```python
from build123d import *

# Parameters (mm, degrees)
SKETCH2_W           = 23
SKETCH2_H           = 10
SKETCH2_R           = 1.05
BOSS_EXTRUDE1_DEPTH = 3
SKETCH3_W           = 10
SKETCH3_H           = 3
BOSS_EXTRUDE2_DEPTH = 25
SKETCH4_R           = 2.1
CUT_EXTRUDE1_DEPTH  = 11
FILLET1_R           = 1.5
FILLET2_R           = 1


with BuildPart() as part:
    # Sketch2 → Boss-Extrude1 (new body)
    with BuildSketch(Plane.XY):
        with Locations((11.5, 5)):
            Rectangle(SKETCH2_W, SKETCH2_H)
        with Locations((4.9, 3)):
            Circle(SKETCH2_R, mode=Mode.SUBTRACT)
        with Locations((18.1, 3)):
            Circle(SKETCH2_R, mode=Mode.SUBTRACT)
    extrude(amount=BOSS_EXTRUDE1_DEPTH)

    # Sketch3 → Boss-Extrude2 (add)
    with BuildSketch(Plane.XY.offset(3)):
        with Locations((11.5, 8.5)):
            Rectangle(SKETCH3_W, SKETCH3_H)
    extrude(amount=-BOSS_EXTRUDE2_DEPTH)

    # Sketch4 → Cut-Extrude1 (cut, through all)
    with BuildSketch(Plane(origin=(0, 10, 0), x_dir=(1, 0, 0), z_dir=(0, 1, 0))):
        with Locations((11.5, 17.5)):
            Circle(SKETCH4_R)
    extrude(amount=-CUT_EXTRUDE1_DEPTH, mode=Mode.SUBTRACT)

    # Fillet1
    fillet1_edges = [part.edges().sort_by_distance(p)[0] for p in [
        (6.5, 8.5, -22),
        (16.5, 8.5, -22),
        (0, 10, 1.5),
        (23, 10, 1.5),
        (23, 0, 1.5),
        (0, 0, 1.5),
    ]]
    fillet(fillet1_edges, radius=FILLET1_R)

    # Fillet2
    fillet2_edges = [part.edges().sort_by_distance(p)[0] for p in [
        (11.5, 7, 0),
        (6.5, 8.5, 0),
        (16.5, 8.5, 0),
    ]]
    fillet(fillet2_edges, radius=FILLET2_R)


solid = part.part
```
Geometry check sheet. Reference: the model listing, model coordinates, mm. A direction names the side the tool comes from. Coordinates: 2 decimals unless noted, no trailing zeros. Order: outer loops, then holes, each group sorted by start corner. A loop starts at its lowest first (then second) coordinate and runs counter-clockwise, first axis right, second up.
Q1. Tool access check on faces 1 (the face through (6.5, 8, -11)), 2 (the face through (17.05, 3.05, 1.48)). Record the directions out of +Z, -Z, +X, -X, +Y, -Y that give a thin tool (end or side, any length) a straight path to the whole face; none if there is none.
Reply:
face 1: -Z, -X, +Y, -Y
face 2: +Z, -Z
Q2. Sectioned sample at D-D on y = 7.5. Record the cut outline in (x, z), and give its area (3 significant figures).
Reply:
outline: (0, 0) - (5.5, 0) arc R1 cw to (6.5, -1) - (6.5, -20.5) arc R1.5 ccw to (8, -22) - (15, -22) arc R1.5 ccw to (16.5, -20.5) - (16.5, -1) arc R1 cw to (17.5, 0) - (23, 0) - (23, 3) - (0, 3) - close; hole circle Ø4.2 at (11.5, -17.5)
area: 275 mm2
Q3. Sectioned sample at A-A on x = 18.1. Record the cut outline in (y, z).
Reply:
outline: (0, 0) - (1.95, 0) - (1.95, 3) - (0, 3) - close; (4.05, 0) - (10, 0) - (10, 3) - (4.05, 3) - close
Q4. Sectioned sample at B-B on z = -17.5. Record the cut outline in (x, y).
Reply:
outline: (6.5, 7) - (9.4, 7) - (9.4, 10) - (6.5, 10) - close; (13.6, 7) - (16.5, 7) - (16.5, 10) - (13.6, 10) - close
Q5. Depth check by flat-ended pin: pin 1 Ø3.5 at (x, z) = (11.5, -17.5) entering from +Y; pin 2 Ø1.5 at (y, z) = (9, -8.5) entering from +X; pin 3 Ø3 at (x, y) = (7.5, 8.5) entering from -Z; pin 4 Ø3 at (x, z) = (13.5, -13) entering from -Y. Enter the tip coordinate at first touch or a pass-through.
Reply:
pin 1: passes through
pin 2: stops at x = 16.5
pin 3: stops at z = -22
pin 4: stops at y = 7
Q6. Sectioned sample at C-C on y = 3. Record the cut outline in (x, z).
Reply:
outline: (0, 0) - (3.85, 0) - (3.85, 3) - (0, 3) - close; (5.95, 0) - (17.05, 0) - (17.05, 3) - (5.95, 3) - close; (19.15, 0) - (23, 0) - (23, 3) - (19.15, 3) - close
Q7. Thickness scan on probe 1 along Y at (x, z) = (4.9, 1.05); probe 2 along Z at (x, y) = (13.5, 2); probe 3 along Z at (x, y) = (11.5, 9.15). Record the ranges inside material, lowest first.
Reply:
probe 1: y = 0 to 1.95, 4.05 to 10
probe 2: z = 0 to 3
probe 3: z = -22 to -19.6, -15.4 to 3
Q8. Draft check along X on faces 3 (the face through (16.5, 8, -11)), 4 (the face through (5.46, 3.89, 1.48)), 5 (the face through (11.584, 6.699, -0.285)). Enter one of: released by +X, released by -X, zero draft, split by the parting line, or undercut.
Reply:
face 3: released by +X
face 4: undercut
face 5: zero draft
